```python
from build123d import *

# Parameters (mm, degrees)
F0_W     = 1257.3
F0_H     = 634.5049866525
F1_DEPTH = 254


# Not quite as in the source:
# - a feature names something its author has since deleted; it is built from what else it names


with BuildPart() as f1:
    # F0 (on Top) → F1 (new body)
    with BuildSketch(Plane.XY):
        with BuildLine():
            ThreePointArc((-425.0103845802, -317.0049866525), (-326.6720587383, -171.8701049425), (-292.1, 0))
            ThreePointArc((-292.1, 0), (-326.8088213402, 172.1959345996), (-425.5148026665, 317.5))
            ThreePointArc((-425.5148026665, 317.5), (-1181.09985954, -0.3533680164), (-425.0103845802, -317.0049866525))
        make_face()
        Polygon((-875.9146199555, 241.3), (-597.2853800445, 241.3), (-457.9707600891, 0), (-597.2853800445, -241.3), (-875.9146199555, -241.3), (-1015.2292399109, 0), align=None, mode=Mode.SUBTRACT)
        with Locations((628.65, 0.2475066738)):
            Rectangle(F0_W, F0_H)
        with BuildLine():
            ThreePointArc((-425.5148026665, 317.5), (-326.8088213402, 172.1959345996), (-292.1, 0))
            ThreePointArc((-292.1, 0), (-326.6720587383, -171.8701049425), (-425.0103845802, -317.0049866525))
            Line((-425.0103845802, -317.0049866525), (0, -317.0049866525))
            Line((0, -317.0049866525), (0, 317.5))
            Line((0, 317.5), (-425.5148026665, 317.5))
        make_face()
    extrude(amount=F1_DEPTH)


solid = f1.part
```
Part model, mm, in its own coordinate system. A direction names the side the tool comes from. Give positions to 0.01 mm unless a question says otherwise; leave off trailing zeros. Write each loop counter-clockwise with the first axis right and the second up, starting at its lowest first coordinate (ties: lowest second). Pieces come first, ordered by that corner, then holes. Notation, with made-up numbers: (57, -28) -> (84, -28) arc R16 ccw to (84, -2) -> close; hole circle Ø4 at (-24, 82.25). An arc over 180 degrees is marked (long way). Put each result on its own line as item: value. Start each with the question number.
Item 1: Cut at D-D (y = 288). List the corners of the cut face in (x, z).
Item 2: Wall check: L1, parallel to Y at x = 668, z = 90; L2, parallel to X at y = -205.5, z = 214.5; L3, parallel to X at y = 155.5, z = 113.5. Give the ranges that are in metal, low to high. Write a range as [from, to].
Item 3: Cut at A-A (x = -736.6). List the corners of the cut face in (y, z), then the cut area to 3 significant figures.
Item 4: Pull direction Y, two halves, no side cores. Call faces 4 (the face through (428, 317.5, 125)), 5 (the face through (-526.653, -118.961, 125.222)), 6 (the face through (21, 6, 0)): pulls with the +Y half, pulls with the -Y half, needs draft (parallel to the pull), parting line crosses it, or undercut.
Item 5: Pin check, flat tips, straight feed: pin 1 Ø6 at (x, z) = (885.5, 152) entering from -Y (3 decimals); pin 2 Ø3 at (y, z) = (-282.5, 134) entering from -X; pin 3 Ø5 at (x, z) = (228.5, 132) entering from +Y. Stop position of each tip, or through.
Item 6: Cut at C-C (y = 35). List the corners of the cut face in (x, z).
Item 7: Which spindle directions (+Z, -Z, +X, -X, +Y, -Y) get a long thin tool onto all of the face, cutting with end or side? Do faces 1 (the face through (21, 6, 254)), 2 (the face through (-946.547, 118.961, 125.222)), 3 (the face through (404, -317.005, 125)). Say none if no direction does.
Item 8: Cut at B-B (z = 222.5). List the corners of the cut face in (x, y), then the cut area to 3 significant figures.
Answer list:
1. outline: (-1075.18, 0) -> (1257.3, 0) -> (1257.3, 254) -> (-1075.18, 254) -> close
2. L1: y = [-317, 317.5]
2. L2: x = [-1130.74, -896.58], [-576.62, 1257.3]
2. L3: x = [-1153.01, -925.45], [-547.75, 1257.3]
3. outline: (-444.5, 0) -> (-241.3, 0) -> (-241.3, 254) -> (-444.5, 254) -> close; (241.3, 0) -> (444.5, 0) -> (444.5, 254) -> (241.3, 254) -> close
3. area: 103,000 mm2
4. face 4: pulls with the +Y half
4. face 5: undercut
4. face 6: needs draft
5. pin 1: stops at y = -317.005
5. pin 2: stops at x = -1081.01
5. pin 3: stops at y = 317.5
6. outline: (-1179.72, 0) -> (-995.02, 0) -> (-995.02, 254) -> (-1179.72, 254) -> close; (-478.18, 0) -> (1257.3, 0) -> (1257.3, 254) -> (-478.18, 254) -> close
7. face 1: +Z, +X, -X, +Y, -Y
7. face 2: +Z, -Z
7. face 3: +Z, -Z, +X, -Y
8. outline: (-425.51, 317.5) arc R444.5 ccw (long way) to (-425.01, -317) -> (1257.3, -317) -> (1257.3, 317.5) -> close; hole (-1015.23, 0) -> (-875.91, -241.3) -> (-597.29, -241.3) -> (-457.97, 0) -> (-597.29, 241.3) -> (-875.91, 241.3) -> close
8. area: 1,430,000 mm2
